Drawing for the job (mm, zero at the part's lowest x, y, z). Round coordinates to 2 decimals unless told otherwise and drop trailing zeros. Write each loop counter-clockwise with the first axis right and the second up, starting at its lowest first coordinate (ties: lowest second). Pieces come first, ordered by that corner, then holes.
Item 1: Band-saw the part on A-A, the plane x = 33.99. Write the cut outline in (y, z).
Item 2: Band-saw the part on C-C, the plane y = 7.5. Write the cut outline in (x, z), then the cut area to 3 significant figures.
Item 3: Band-saw the part on B-B, the plane z = 33.99. Write the cut outline in (x, y), then the cut area to 3 significant figures.
Item 4: Drop flat-ended pins along their axis: pin 1 Ø5 at (y, z) = (5, 37) entering from -X; pin 2 Ø2 at (y, z) = (9, 34) entering from +X; pin 3 Ø3 at (y, z) = (8, 22.5) entering from -X. Give the stop position or say it passes through.
Item 5: Wall check: probe 1 along X at (y, z) = (4, 33.99); probe 2 along X at (y, z) = (1.5, 6.5); probe 3 along X at (y, z) = (3.5, 52). Give the ranges that are in metal, low to high.
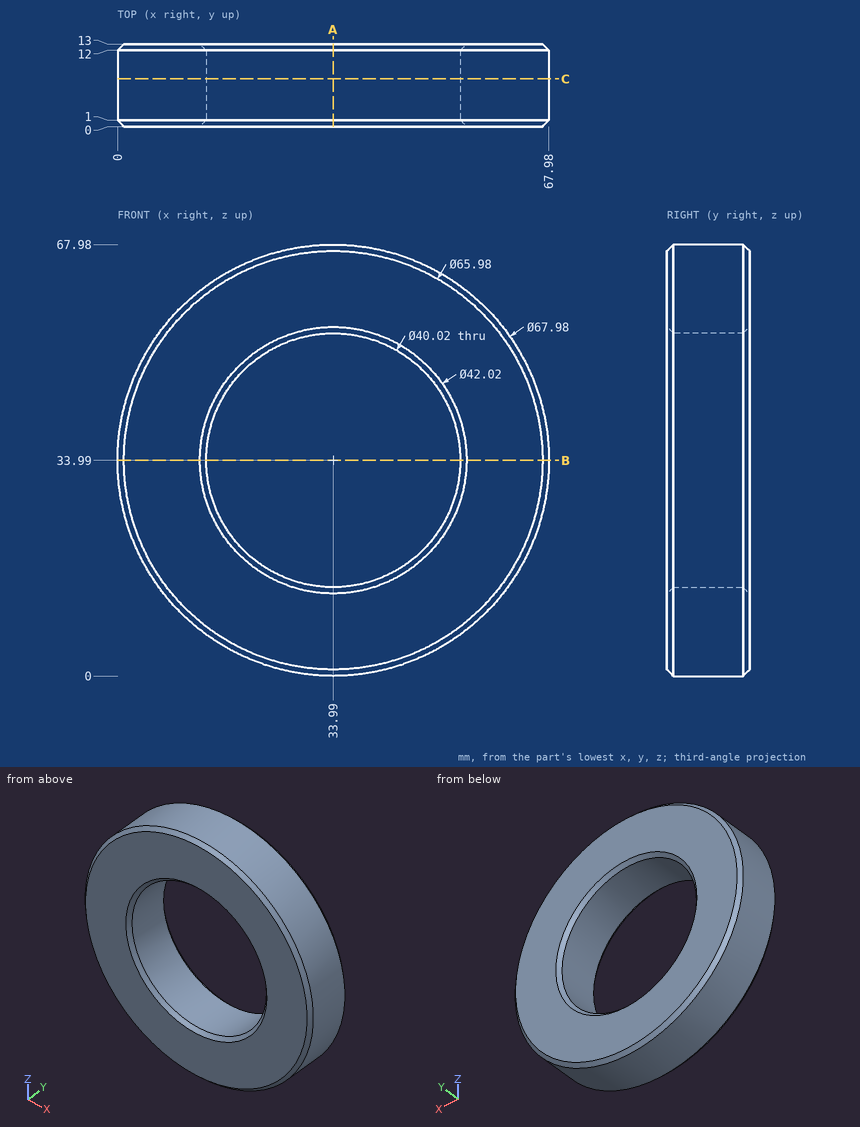
Results:
1. outline: (0, 1) - (1, 0) - (12, 0) - (13, 1) - (13, 12.98) - (12, 13.98) - (1, 13.98) - (0, 12.98) - close; (0, 55) - (1, 54) - (12, 54) - (13, 55) - (13, 66.98) - (12, 67.98) - (1, 67.98) - (0, 66.98) - close
2. outline: circle Ø67.98 at (33.99, 33.99); hole circle Ø40.02 at (33.99, 33.99)
2. area: 2,370 mm2
3. outline: (0, 1) - (1, 0) - (12.98, 0) - (13.98, 1) - (13.98, 12) - (12.98, 13) - (1, 13) - (0, 12) - close; (54, 1) - (55, 0) - (66.98, 0) - (67.98, 1) - (67.98, 12) - (66.98, 13) - (55, 13) - (54, 12) - close
3. area: 359 mm2
4. pin 1: stops at x = 0
4. pin 2: stops at x = 67.98
4. pin 3: stops at x = 1.5
5. probe 1: x = 0 to 13.98, 54 to 67.98
5. probe 2: x = 14 to 53.98
5. probe 3: x = 5.16 to 25.27, 42.71 to 62.82
